Geometry check sheet. Reference: the model listing, model coordinates, mm. A direction names the side the tool comes from. Give positions to 0.01 mm unless a question says otherwise; leave off trailing zeros. Loops run counter-clockwise (first coordinate to the right, second up) from the corner with the lowest first, then second, coordinate; pieces in that order, holes last. Notation, with made-up numbers: (-1, 67.25) -> (39, 67.25) arc R17 ccw to (39, 99.25) -> close; hole circle Ø3 at (36.25, 55). An arc over 180 degrees is marked (long way). Answer in a Markdown table with one row per item. Add a question column.
```python
from build123d import *

# Parameters (mm, degrees)
PAD_DEPTH    = 10
FILLET_R     = 3
SKETCH001_R  = 1.7
POCKET_DEPTH = 56.501


with BuildPart() as part:
    # Sketch → Pad (new body)
    with BuildSketch(Plane.YZ):
        with BuildLine():
            ThreePointArc((-13.774977, 2.5), (0, -14), (13.774977, 2.5))
            Line((8.124038, 37.5), (13.774977, 2.5))
            Line((10.198039, 37.5), (8.124038, 37.5))
            Line((10.198039, 37.5), (15.803481, 2.5))
            Line((15.803481, 2.5), (15.803481, -19))
            Line((-15.803481, -19), (15.803481, -19))
            Line((-15.803481, 2.5), (-15.803481, -19))
            Line((-15.803481, 2.5), (-10.198039, 37.5))
            Line((-8.124038, 37.5), (-10.198039, 37.5))
            Line((-13.774977, 2.5), (-8.124038, 37.5))
        make_face()
    extrude(amount=PAD_DEPTH)

    # Fillet
    fillet_edges = [part.edges().sort_by_distance(p)[0] for p in [
        (5, -15.803481, -19),
        (5, 15.803481, -19),
    ]]
    fillet(fillet_edges, radius=FILLET_R)

    # Sketch001 (on Face6 of Fillet) → Pocket (cut, through all)
    with BuildSketch(Plane.YX.offset(19)):
        with Locations((0, 5)):
            Circle(SKETCH001_R)
    extrude(amount=-POCKET_DEPTH, mode=Mode.SUBTRACT)


solid = part.part
```
1. Material ranges on L1, parallel to Y at x = 5.25, z = 0; L2, parallel to X at y = 0, z = -17.8; L3, parallel to Y at x = 5, z = -15.5, recorded low to high. Write a range as from..to.
2. Gauge pin test, flat end, axial feed: pin 1 Ø4 at (x, z) = (4, 6.5) entering from +Y. Record the tip position at first contact, or that the pin passes through.
3. Sectioned sample at C-C (x = 5). Enter the section's corners in (y, z).
4. Release check for a two-part mould opening along Z. For faces 1 (the face through (5, 9, 37.5)), 2 (the face through (4.93, 10.91, 20.24)), 3 (the face through (5, 15.803, -7)) record: released by +Z, released by -Z, zero draft, split by the parting line, or undercut.
5. Sectioned sample at A-A (z = 0). Enter the section's corners in (x, y), plus the area to 3 significant figures.
6. Access from +Z, -Z, +X, -X, +Y, -Y to the whole of each face (thin tool, end or side, straight path). Record for faces 4 (the face through (4.93, -10.99, 19.76)), 5 (the face through (5, -15.803, -7)).
7. Sectioned sample at B-B (y = 0). Enter the section's corners in (x, z).
Response:
| question | item | result |
|---|---|---|
| 1 | L1 | y = -15.8..-14, 14..15.8 |
| 1 | L2 | x = 0..3.3, 6.7..10 |
| 1 | L3 | y = -15.8..-1.7, 1.7..15.8 |
| 2 | pin 1 | stops at y = 15.48 |
| 3 | outline | (-15.8, -16) arc R3 ccw to (-12.8, -19) -> (-1.7, -19) -> (-1.7, -13.9) arc R14 cw to (-13.77, 2.5) -> (-8.12, 37.5) -> (-10.2, 37.5) -> (-15.8, 2.5) -> close; (1.7, -19) -> (12.8, -19) arc R3 ccw to (15.8, -16) -> (15.8, 2.5) -> (10.2, 37.5) -> (8.12, 37.5) -> (13.77, 2.5) arc R14 cw to (1.7, -13.9) -> close |
| 4 | face 1 | released by +Z |
| 4 | face 2 | undercut |
| 4 | face 3 | zero draft |
| 5 | outline | (0, -15.8) -> (10, -15.8) -> (10, -14) -> (0, -14) -> close; (0, 14) -> (10, 14) -> (10, 15.8) -> (0, 15.8) -> close |
| 5 | area | 36.1 mm2 |
| 6 | face 4 | +X, -X |
| 6 | face 5 | +Z, -Z, +X, -X, -Y |
| 7 | outline | (0, -19) -> (3.3, -19) -> (3.3, -14) -> (0, -14) -> close; (6.7, -19) -> (10, -19) -> (10, -14) -> (6.7, -14) -> close |
